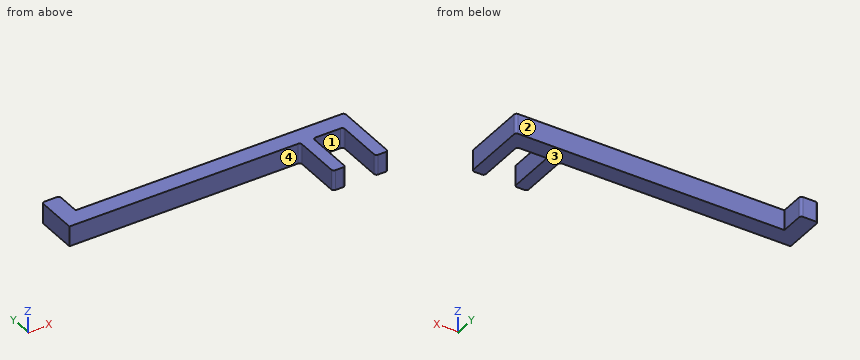
```python
from build123d import *

# Parameters (mm, degrees)
EXTRUDE_1_DEPTH     = 12
CUT_EXTRUDE_1_DEPTH = 82


with BuildPart() as part:
    # Эскиз1 → Бобышка-Вытянуть1 (new body)
    with BuildSketch(Plane.XY):
        with BuildLine():
            Line((-47.73428915, 17), (-42.73428915, 17))
            ThreePointArc((-42.73428915, 17), (-42.027182368, 16.707106781), (-41.73428915, 16))
            Line((-41.73428915, 16), (-41.73428915, 7))
            Line((-41.73428915, 7), (25.229943888, 7))
            Line((25.229943888, 7), (64.26571085, 7))
            ThreePointArc((64.26571085, 7), (64.972817632, 6.707106781), (65.26571085, 6))
            Line((65.26571085, 6), (65.26571085, -19))
            ThreePointArc((65.26571085, -19), (64.972817632, -19.707106781), (64.26571085, -20))
            Line((64.26571085, -20), (61.26571085, -20))
            ThreePointArc((61.26571085, -20), (60.558604069, -19.707106781), (60.26571085, -19))
            Line((60.26571085, -19), (60.26571085, -1))
            ThreePointArc((60.26571085, -1), (59.972817632, -0.292893219), (59.26571085, 0))
            Line((59.26571085, 0), (49.26571085, 0))
            ThreePointArc((49.26571085, 0), (48.558604069, -0.292893219), (48.26571085, -1))
            Line((48.26571085, -1), (48.26571085, -19))
            ThreePointArc((48.26571085, -19), (47.972817632, -19.707106781), (47.26571085, -20))
            Line((47.26571085, -20), (44.26571085, -20))
            ThreePointArc((44.26571085, -20), (43.558604069, -19.707106781), (43.26571085, -19))
            Line((43.26571085, -19), (43.26571085, -1))
            ThreePointArc((43.26571085, -1), (42.972817632, -0.292893219), (42.26571085, 0))
            Line((42.26571085, 0), (-48.73428915, 0))
            Line((-48.73428915, 0), (-48.73428915, 16))
            ThreePointArc((-48.73428915, 16), (-48.441395931, 16.707106781), (-47.73428915, 17))
        make_face()
    extrude(amount=EXTRUDE_1_DEPTH)

    # Эскиз2 → Вырез-Вытянуть1 (cut)
    with BuildSketch(Plane(origin=(0, 17, 0), x_dir=(1, 0, 0), z_dir=(0, 1, 0))):
        Polygon((81.423814873, -4), (-154.472854851, -4), (-146.348766817, 32.606222342), (92.957474686, 29.235711898), align=None)
        Polygon((81.423814873, -16), (-154.472854851, -16), (-172.112104827, -50.666366553), (103.309756763, -54.545547702), align=None)
    extrude(amount=-CUT_EXTRUDE_1_DEPTH, mode=Mode.SUBTRACT)


solid = part.part
```
The listing builds one solid part. Answer for the finished solid, in the listing's coordinates (mm). Face numbers are marked on the shaded views. A direction names the side the tool comes from. Round coordinates to 2 decimals unless told otherwise and drop trailing zeros. Loops run counter-clockwise (first coordinate to the right, second up) from the corner with the lowest first, then second, coordinate; pieces in that order, holes last. Notation, with made-up numbers: (31, -16) - (36, -16) arc R23 cw to (36, 14) - close; hole circle Ø3 at (89.25, 22). An arc over 180 degrees is marked (long way). Return JSON: item names as keys, results as strings. Group by question number.
1. The mould has two halves that part along X. Classify the marked faces 1 and 2: pulls with the +X half, pulls with the -X half, needs draft (parallel to the pull), parting line crosses it, or undercut.
2. Which of the six approach directions +Z, -Z, +X, -X, +Y, -Y give full straight-line access (tool end or side, diameter ignored) to the marked faces 3 and 4?
3. The part is cut by section A-A on z = 10.75. Determine the outline of the cut face in (x, y).
4. Each of these flat-tipped pins is pushed along its axis until it touches: P1, Ø4, axis at x = -4, z = 7, coming from the -Y side; P2, Ø4, axis at y = -12.5, z = 7.5, coming from the -X side; P3, Ø2, axis at x = 2, z = 8.5, coming from the +Y side. Where does it stop, or does it pass through?
5. The part is cut by section B-B on y = 10. Determine the outline of the cut face in (x, z), then the cut area to 3 significant figures.
6. The part is cut by section C-C on x = -37. Determine the outline of the cut face in (y, z).
7. Consider probe 1 along X at (y, z) = (-16, 4.5); probe 2 along Y at (x, z) = (-24, 10.75); probe 3 along X at (y, z) = (9, 9). Determine where each line is inside the solid, lowest interval first.
Resolved:
{
 "1": {"face 1": "undercut", "face 2": "needs draft"},
 "2": {"face 3": "-Z, +X, -X, +Y, -Y", "face 4": "+Z, -Z, -X, -Y"},
 "3": {"outline": "(-48.73, 0) - (42.27, 0) arc R1 cw to (43.27, -1) - (43.27, -19) arc R1 ccw to (44.27, -20) - (47.27, -20) arc R1 ccw to (48.27, -19) - (48.27, -1) arc R1 cw to (49.27, 0) - (59.27, 0) arc R1 cw to (60.27, -1) - (60.27, -19) arc R1 ccw to (61.27, -20) - (64.27, -20) arc R1 ccw to (65.27, -19) - (65.27, 6) arc R1 ccw to (64.27, 7) - (-41.73, 7) - (-41.73, 16) arc R1 ccw to (-42.73, 17) - (-47.73, 17) arc R1 ccw to (-48.73, 16) - close"},
 "4": {"P1": "stops at y = 0", "P2": "stops at x = 43.27", "P3": "stops at y = 7"},
 "5": {"outline": "(-48.73, 4) - (-41.73, 4) - (-41.73, 12) - (-48.73, 12) - close", "area": "56.0 mm²"},
 "6": {"outline": "(0, 4) - (7, 4) - (7, 12) - (0, 12) - close"},
 "7": {"probe 1": "x = 43.27 to 48.27, 60.27 to 65.27", "probe 2": "y = 0 to 7", "probe 3": "x = -48.73 to -41.73"}
}
